The figure shows three views and two pictorial views of one solid part (mm, origin at its lowest corner). Answer the questions. Round coordinates to 2 decimals unless told otherwise and drop trailing zeros. Loops run counter-clockwise (first coordinate to the right, second up) from the corner with the lowest first, then second, coordinate; pieces in that order, holes last. Notation, with made-up numbers: (81.25, 37) -> (117.25, 37) arc R14 cw to (117.25, 47) -> close; hole circle Ø6 at (55.5, 54). An arc over 180 degrees is marked (long way). Put each result on its own line as item: value.
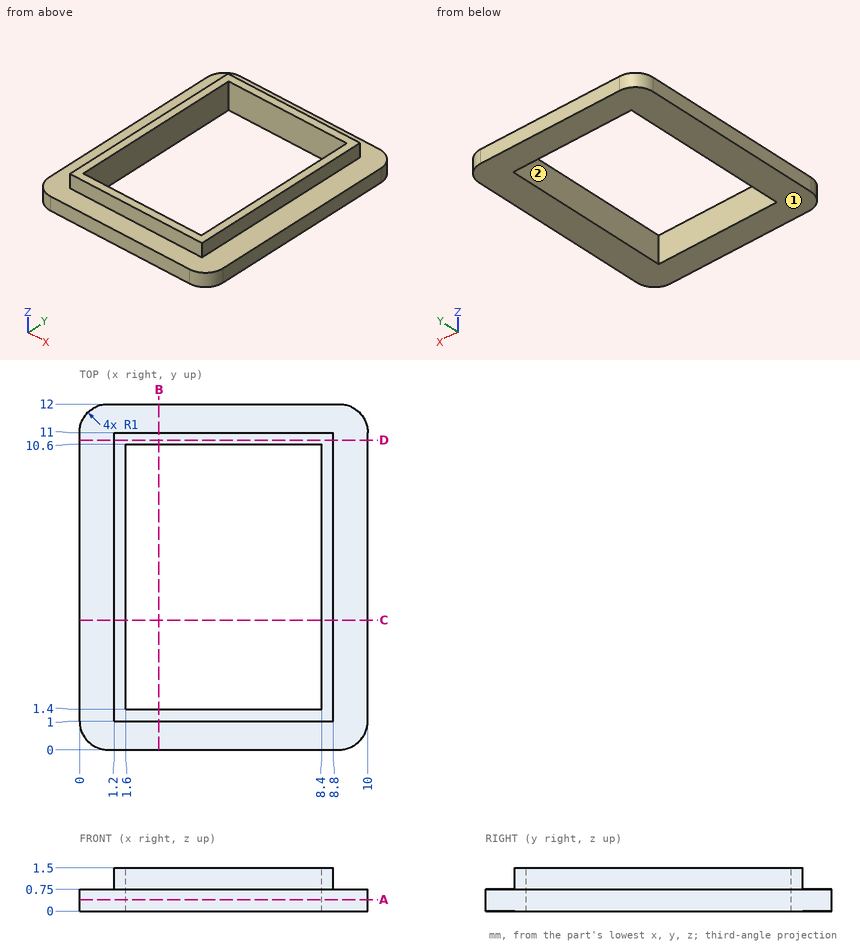
Item 1: The part is cut by section D-D (y = 10.75). Determine the outline of the cut face in (x, z).
Derived:
outline: (0, 0) -> (10, 0) -> (10, 0.75) -> (8.8, 0.75) -> (8.8, 1.5) -> (1.2, 1.5) -> (1.2, 0.75) -> (0, 0.75) -> close
Item 2: The part is cut by section B-B (x = 2.75). Determine the outline of the cut face in (y, z), then the cut area to 3 significant figures.
Derived:
outline: (0, 0) -> (1.4, 0) -> (1.4, 1.5) -> (1, 1.5) -> (1, 0.75) -> (0, 0.75) -> close; (10.6, 0) -> (12, 0) -> (12, 0.75) -> (11, 0.75) -> (11, 1.5) -> (10.6, 1.5) -> close
area: 2.70 mm^2
Item 3: For a pull along Y with two mould halves and no side action, classify the marked faces 1 and 2 as pulls with the +Y half, pulls with the -Y half, needs draft (parallel to the pull), parting line crosses it, or undercut.
Derived:
face 1: needs draft
face 2: undercut
Item 4: Find the intervals of material crossed by line 1 along Y through (x, z) = (8, 0.9); line 2 along X through (y, z) = (1.75, 1.1); line 3 along X through (y, z) = (5.25, 0.55), in increasing order.
Derived:
line 1: y = 1 to 1.4, 10.6 to 11
line 2: x = 1.2 to 1.6, 8.4 to 8.8
line 3: x = 0 to 1.6, 8.4 to 10
Item 5: The part is cut by section A-A (z = 0.4). Determine the outline of the cut face in (x, y), then the cut area to 3 significant figures.
Derived:
outline: (0, 1) arc R1 ccw to (1, 0) -> (9, 0) arc R1 ccw to (10, 1) -> (10, 11) arc R1 ccw to (9, 12) -> (1, 12) arc R1 ccw to (0, 11) -> close; hole (1.6, 1.4) -> (8.4, 1.4) -> (8.4, 10.6) -> (1.6, 10.6) -> close
area: 56.6 mm^2
Item 6: Flat-ended cylindrical pins translate along their axes: pin 1 Ø0.8 at (x, z) = (5, 1.5) entering from +Y; pin 2 Ø4 at (x, y) = (5.5, 8) entering from +Z. Find the tip coordinate at first contact, or state that the pin passes through.
Derived:
pin 1: stops at y = 11
pin 2: passes through
Item 7: The part is cut by section C-C (y = 4.5). Determine the outline of the cut face in (x, z), then the cut area to 3 significant figures.
Derived:
outline: (0, 0) -> (1.6, 0) -> (1.6, 1.5) -> (1.2, 1.5) -> (1.2, 0.75) -> (0, 0.75) -> close; (8.4, 0) -> (10, 0) -> (10, 0.75) -> (8.8, 0.75) -> (8.8, 1.5) -> (8.4, 1.5) -> close
area: 3.00 mm^2
